```python
from build123d import *

# Parameters (mm, degrees)
SKETCH1_W                                      = 124.8
SKETCH1_H                                      = 50.9
SKETCH1_W_2                                    = 12.6
SKETCH1_H_2                                    = 12.1
BOSS_EXTRUDE1_DEPTH                            = 1.45
CSK_FOR_M3_5_FLAT_HEAD_MACHINE_SCREW1_AT_COUNT = 2
CSK_FOR_M3_5_FLAT_HEAD_MACHINE_SCREW1_AT_PITCH = 115.5
CSK_FOR_M3_5_FLAT_HEAD_MACHINE_SCREW_2_COUNT   = 2
CSK_FOR_M3_5_FLAT_HEAD_MACHINE_SCREW_2_PITCH   = 123.420014584
CSK_FOR_M3_5_FLAT_HEAD_MACHINE_SCREW_3_COUNT   = 2
CSK_FOR_M3_5_FLAT_HEAD_MACHINE_SCREW_3_PITCH   = 43.5
FILLET2_R                                      = 4


with BuildPart() as part:
    # Sketch1 → Boss-Extrude1 (new body)
    with BuildSketch(Plane.XY):
        with Locations((62.4, -25.45)):
            Rectangle(SKETCH1_W, SKETCH1_H)
        with Locations((37.585, -19.035)):
            Rectangle(SKETCH1_W_2, SKETCH1_H_2, mode=Mode.SUBTRACT)
    extrude(amount=BOSS_EXTRUDE1_DEPTH)

    # Sketch2 → CSK for M3.5 Flat Head Machine Screw1 (revolve, cut)
    with BuildSketch(Plane(origin=(4.65, -3.7, 1.45), x_dir=(0, -1, 0), z_dir=(1, 0, 0))):
        Polygon((0, 0), (0, 1.45), (1.75, 1.45), (1.75, 1.294164458), (2.875, 0), align=None)
    csk_for_m3_5_flat_head_machine_screw1 = revolve(axis=Axis((4.65, -3.7, 7.8), (0, 0, -1)), mode=Mode.SUBTRACT)

    # CSK for M3.5 Flat Head Machine Screw1 at: CSK for M3.5 Flat Head Machine Screw1 ×2
    with Locations(*[(i * CSK_FOR_M3_5_FLAT_HEAD_MACHINE_SCREW1_AT_PITCH, 0, 0) for i in range(1, CSK_FOR_M3_5_FLAT_HEAD_MACHINE_SCREW1_AT_COUNT)]):
        add(csk_for_m3_5_flat_head_machine_screw1, mode=Mode.SUBTRACT)

    # CSK for M3.5 Flat Head Machine Screw 2: CSK for M3.5 Flat Head Machine Screw1 ×2
    with Locations(*[Vector(0.935828766, -0.35245499, 0) * (i * CSK_FOR_M3_5_FLAT_HEAD_MACHINE_SCREW_2_PITCH) for i in range(1, CSK_FOR_M3_5_FLAT_HEAD_MACHINE_SCREW_2_COUNT)]):
        add(csk_for_m3_5_flat_head_machine_screw1, mode=Mode.SUBTRACT)

    # CSK for M3.5 Flat Head Machine Screw 3: CSK for M3.5 Flat Head Machine Screw1 ×2
    with Locations(*[(0, -i * CSK_FOR_M3_5_FLAT_HEAD_MACHINE_SCREW_3_PITCH, 0) for i in range(1, CSK_FOR_M3_5_FLAT_HEAD_MACHINE_SCREW_3_COUNT)]):
        add(csk_for_m3_5_flat_head_machine_screw1, mode=Mode.SUBTRACT)

    # Fillet2
    fillet2_edges = [part.edges().sort_by_distance(p)[0] for p in [
        (124.8, -50.9, 0.725),
        (0, -50.9, 0.725),
        (0, 0, 0.725),
        (124.8, 0, 0.725),
    ]]
    fillet(fillet2_edges, radius=FILLET2_R)


solid = part.part
```
Read the model definition and answer for the solid it produces. Units are mm, in the model's axes. Round coordinates to 2 decimals unless told otherwise and drop trailing zeros. Loops run counter-clockwise (first coordinate to the right, second up) from the corner with the lowest first, then second, coordinate; pieces in that order, holes last. Notation, with made-up numbers: (41, -6.75) -> (77, -6.75) arc R19 ccw to (77, 18.25) -> close; hole circle Ø1 at (-27, 17.25). An arc over 180 degrees is marked (long way). One line per item, written item: value.
1) A flat-ended cylindrical pin translates along its axis: P1, Ø3, axis at x = 4.65, y = -47.2, coming from the -Z side. Find the tip coordinate at first contact, or state that the pin passes through.
Answer list:
P1: passes through
2) Consider L1, parallel to Y at x = 4.65, z = 0.15; L2, parallel to X at y = -3.7, z = 0.1; L3, parallel to X at y = -18, z = 1.3 (3 decimals). Determine where each line is inside the solid, lowest interval first. Write a range as [from, to].
Answer list:
L1: y = [-50.9, -48.95], [-45.45, -5.45], [-1.95, 0]
L2: x = [0.01, 2.9], [6.4, 118.4], [121.9, 124.79]
L3: x = [0, 31.285], [43.885, 124.8]
3) The mould has two halves that part along X. Classify faces 1 (the face through (123.597, -49.759, 0.735)), 2 (the face through (1.141, -1.203, 0.735)), 3 (the face through (62, -25, 1.45)): pulls with the +X half, pulls with the -X half, needs draft (parallel to the pull), parting line crosses it, or undercut.
Answer list:
face 1: pulls with the +X half
face 2: pulls with the -X half
face 3: needs draft
4) A cutting plane is placed at B-B (y = -22). Determine the outline of the cut face in (x, z) (3 decimals).
Answer list:
outline: (0, 0) -> (31.285, 0) -> (31.285, 1.45) -> (0, 1.45) -> close; (43.885, 0) -> (124.8, 0) -> (124.8, 1.45) -> (43.885, 1.45) -> close
5) A cutting plane is placed at A-A (x = 36). Determine the outline of the cut face in (y, z) (3 decimals).
Answer list:
outline: (-50.9, 0) -> (-25.085, 0) -> (-25.085, 1.45) -> (-50.9, 1.45) -> close; (-12.985, 0) -> (0, 0) -> (0, 1.45) -> (-12.985, 1.45) -> close
6) A cutting plane is placed at C-C (z = 0.65). Determine the outline of the cut face in (x, y) (3 decimals).
Answer list:
outline: (0, -46.9) arc R4 ccw to (4, -50.9) -> (120.8, -50.9) arc R4 ccw to (124.8, -46.9) -> (124.8, -4) arc R4 ccw to (120.8, 0) -> (4, 0) arc R4 ccw to (0, -4) -> close; hole circle Ø4.359 at (4.65, -47.2); hole circle Ø4.359 at (4.65, -3.7); hole (31.285, -25.085) -> (43.885, -25.085) -> (43.885, -12.985) -> (31.285, -12.985) -> close; hole circle Ø4.359 at (120.15, -47.2); hole circle Ø4.359 at (120.15, -3.7)
